The listing builds one solid part. Answer for the finished solid, in the listing's coordinates (mm). A direction names the side the tool comes from. Coordinates: 2 decimals unless noted, no trailing zeros. Write each loop counter-clockwise with the first axis right and the second up, starting at its lowest first coordinate (ties: lowest second). Pieces come first, ordered by that corner, then holes.
(1) For a pull along Y with two mould halves and no side action, classify faces 1 (the flat face through (-18, -13, 0)), 2 (the flat face through (17, -14, 4.9)), 3 (the flat face through (16, -14, 6.7)), 4 (the cylindrical face through (-17.427, 14.005, 8.921)) as +Y half, -Y half, draft (parallel to the pull), parting line (faces both ways), or undercut.
(2) Which of the six approach directions +Z, -Z, +X, -X, +Y, -Y give full straight-line access (tool end or side, diameter ignored) to faces 5 (the flat face through (16, -14, 6.2)), 6 (the flat face through (19.548, -14, 4))?
(3) The part is cut by section B-B on z = 2.25. Determine the outline of the cut face in (x, y), plus the area to 3 significant figures.
(4) Straight lines are drawn through the part: line 1 (Y direction, x = -45.5, z = 5.5); line 2 (Y direction, x = -19, z = 3.25); line 3 (Z direction, x = 7, y = -39). For each, find the intervals that lie inside material, in ascending order.
(5) Given P1, Ø0.6, axis at y = -12.5, z = 6.5, coming from the +X side, flat-ended and moving along its own axis, determine where the tip first touches the part or whether it passes through.
from build123d import *

# Parameters (mm, degrees)
F0_W     = 75
F0_H     = 58
F1_DEPTH = 10.5
F3_R     = 5.24999
F4_DEPTH = 6
F5_W     = 6.9
F5_H     = 0.25
F6_DEPTH = 4.572
F7_R     = 0.24999


# Not quite as in the source:
# - a fillet or chamfer is up to 0.001 mm smaller than in the source, because OpenCascade refuses the exact size


with BuildPart() as f1:
    # F0 (on Top) → F1 (new body)
    with BuildSketch(Plane.XY):
        with Locations((-17.9516240954, -13.4977242947)):
            Rectangle(F0_W, F0_H)
    extrude(amount=F1_DEPTH)

    # F3 (radius 5.25 in the source; OpenCascade refuses exactly that, so slightly less here)
    f3_edges = [f1.edges().sort_by_distance(p)[0] for p in [
        (-17.951624, -42.497724, 10.5),
        (-17.951624, -42.497724, 0),
        (-17.951624, 15.502276, 10.5),
        (-17.951624, 15.502276, 0),
    ]]
    fillet(f3_edges, radius=F3_R)

    # F2 (on face) → F4 (cut)
    with BuildSketch(Plane.YZ.offset(19.5483759046)):
        with BuildLine():
            Line((-10.0477242947, 8), (-13.4977242947, 8))
            Line((-13.4977242947, 8), (-16.9477242947, 8))
            ThreePointArc((-16.9477242947, 8), (-15.8517087838, 7.5460155108), (-15.3977242947, 6.45))
            ThreePointArc((-15.3977242947, 6.45), (-15.8517087838, 5.3539844892), (-16.9477242947, 4.9))
            Line((-16.9477242947, 4.9), (-10.0477242947, 4.9))
            ThreePointArc((-10.0477242947, 4.9), (-11.5977242947, 6.45), (-10.0477242947, 8))
        make_face()
        with BuildLine():
            Line((-10.0477242947, 4.9), (-10.0477242947, 8))
            ThreePointArc((-10.0477242947, 8), (-11.5977242947, 6.45), (-10.0477242947, 4.9))
        make_face()
        with BuildLine():
            ThreePointArc((-8.4977242947, 6.45), (-8.9517087838, 7.5460155108), (-10.0477242947, 8))
            Line((-10.0477242947, 8), (-10.0477242947, 4.9))
            ThreePointArc((-10.0477242947, 4.9), (-8.9517087838, 5.3539844892), (-8.4977242947, 6.45))
        make_face()
        with BuildLine():
            ThreePointArc((-15.3977242947, 6.45), (-15.8517087838, 7.5460155108), (-16.9477242947, 8))
            Line((-16.9477242947, 8), (-16.9477242947, 4.9))
            ThreePointArc((-16.9477242947, 4.9), (-15.8517087838, 5.3539844892), (-15.3977242947, 6.45))
        make_face()
        with BuildLine():
            Line((-16.9477242947, 4.9), (-16.9477242947, 8))
            ThreePointArc((-16.9477242947, 8), (-18.0437398055, 7.5460155108), (-18.4977242947, 6.45))
            ThreePointArc((-18.4977242947, 6.45), (-18.0437398055, 5.3539844892), (-16.9477242947, 4.9))
        make_face()
    extrude(amount=-F4_DEPTH, mode=Mode.SUBTRACT)

    # F5 (on face) → F6 (join)
    with BuildSketch(Plane.YZ.offset(13.5483759046)):
        with Locations((-13.4977242947, 6.575)):
            Rectangle(F5_W, F5_H)
        with Locations((-13.4977242947, 6.325)):
            Rectangle(F5_W, F5_H)
    extrude(amount=F6_DEPTH)

    # F7 (radius 0.25 in the source; OpenCascade refuses exactly that, so slightly less here)
    f7_edges = [f1.edges().sort_by_distance(p)[0] for p in [
        (15.834376, -10.047724, 6.7),
        (15.834376, -10.047724, 6.2),
        (15.834376, -16.947724, 6.7),
        (15.834376, -16.947724, 6.2),
    ]]
    fillet(f7_edges, radius=F7_R)


solid = f1.part
Model answer:
1. face 1: draft
1. face 2: undercut
1. face 3: undercut
1. face 4: +Y half
2. face 5: +X
2. face 6: +Z, -Z, +X, +Y, -Y
3. outline: (-55.45, -41.56) - (19.55, -41.56) - (19.55, 14.56) - (-55.45, 14.56) - close
3. area: 4,210 mm2
4. line 1: y = -42.49 to 15.5
4. line 2: y = -42.1 to 15.11
4. line 3: z = 0.3 to 10.2
5. P1: stops at x = 18.12
